Could you check a few things on this model? Use its own coordinates, in mm. Face numbers are marked on the shaded views. A direction names the side the tool comes from. Give positions to 0.01 mm unless a question says otherwise; leave off trailing zeros. Loops run counter-clockwise (first coordinate to the right, second up) from the corner with the lowest first, then second, coordinate; pieces in that order, holes last. Notation, with made-up numbers: (-13.75, 70.25) - (1.25, 70.25) arc R17 cw to (1.25, 84.25) - close; hole circle Ø7 at (62, 53). An arc over 180 degrees is marked (long way). Use CSV: the item, a comma, the result in double quotes.
from build123d import *

# Parameters (mm, degrees)
F_3_8_0_375_DIAMETER_HOLE1_D = 9.525
F_3_8_CLEARANCE_HOLE1_D      = 10.0838
CIRPATTERN1_COUNT            = 6


with BuildPart() as part:
    # Sketch1 → Revolve1 (revolve)
    with BuildSketch(Plane.XY):
        Polygon((-12.827, 0), (-50.8, 0), (-50.8, 12.7), (-19.05, 12.7), (-19.05, 38.1), (0, 38.1), (0, 0), (-9.525, 0), (-9.525, 2.54), (-12.827, 2.54), align=None)
    revolve(axis=Axis((0, 38.1, 0), (0, -1, 0)))

    # 3/8 (0.375) Diameter Hole1 (through all)
    with Locations(Plane(origin=(0, 38.1, 0), x_dir=(1, 0, 0), z_dir=(0, 1, 0))):
        with Locations((0, 0)):
            Hole(F_3_8_0_375_DIAMETER_HOLE1_D / 2)

    # Sketch3 → 1/2 NPT Tapped Hole1 (revolve, cut)
    with BuildSketch(Plane(origin=(0, 38.1, 0), x_dir=(0, 0, 1), z_dir=(1, 0, 0))):
        Polygon((0, 0), (0, 27.970543693), (8.9281, 22.606), (8.9281, 13.462), (9.479726792, 13.462), (9.8827971, 0), align=None)
    revolve(axis=Axis((0, 44.45, 0), (0, -1, 0)), mode=Mode.SUBTRACT)

    # 3/8 Clearance Hole1 (through all)
    with Locations(Plane(origin=(0, 12.7, 0), x_dir=(1, 0, 0), z_dir=(0, 1, 0))):
        with Locations((38.1, 0)):
            f_3_8_clearance_hole1 = Hole(F_3_8_CLEARANCE_HOLE1_D / 2)

    # CirPattern1: 3/8 Clearance Hole1 ×6 about axis
    cirpattern1_axis = Axis((0, 0, 0), (0, 1, 0))
    for i in range(1, CIRPATTERN1_COUNT):
        add(f_3_8_clearance_hole1.rotate(cirpattern1_axis, i * 360 / CIRPATTERN1_COUNT), mode=Mode.SUBTRACT)


solid = part.part
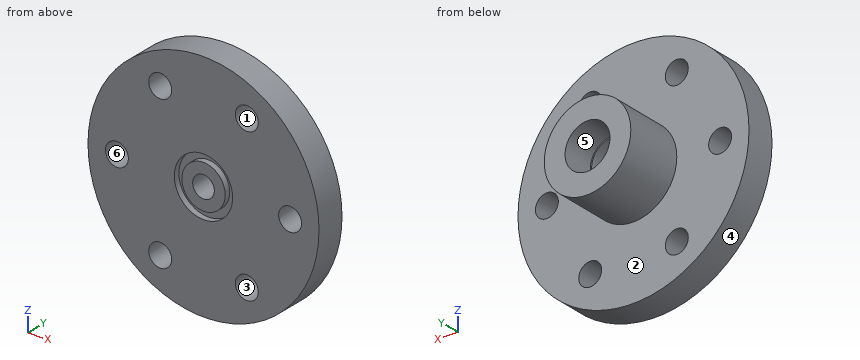
1) Which directions (+Z, -Z, +X, -X, +Y, -Y) give clear straight access to the entire face, cutting with the end or side of a thin tool? Please do the marked faces 5 and 6.
Answer below:
face 5,"+Y"
face 6,"+Y, -Y"
2) Suppose I cut it at B-B (x = 38.1). Please give me the cut outline in (y, z).
Answer below:
outline,"(0, -33.6) - (12.7, -33.6) - (12.7, -5.04) - (0, -5.04) - close; (0, 5.04) - (12.7, 5.04) - (12.7, 33.6) - (0, 33.6) - close"
3) We'd pull the mould along X, two halves only. Please class the marked faces 1, 2, 3 and 4: +X half, -X half, draft (parallel to the pull), parting line (faces both ways), or undercut.
Answer below:
face 1,"undercut"
face 2,"draft"
face 3,"undercut"
face 4,"parting line"
4) Suppose I cut it at D-D (z = -2). State how many separate pieces and enclosed holes the cut face has, plus the area to 3 significant figures.
Answer below:
separate pieces,"4"
enclosed holes,"0"
area,"1,440 mm2"
5) I'm going to push flat-ended pins straight in: P1, Ø9, axis at x = -38.1, z = 0, coming from the +Y side; P2, Ø11.5, axis at x = -19.05, z = 33, coming from the +Y side; P3, Ø1, axis at x = -9, y = 24, coming from the +Z side; P4, Ø1, axis at x = -2.5, y = 25, coming from the +Z side. Where does each tip first touch, or does it pass through?
Answer below:
P1,"passes through"
P2,"stops at y = 12.7"
P3,"stops at z = 17.05"
P4,"stops at z = 18.94"
6) I need wall thicknesses on line 1 along Z through (x, y) = (0, 17); line 2 along Z through (x, y) = (-19.05, 4); line 3 along Z through (x, y) = (0, 6). Which ranges of each line are inside material? Lowest first, please.
Answer below:
line 1,"z = -19.05 to -8.93, 8.93 to 19.05"
line 2,"z = -47.09 to -38.04, -27.95 to 27.95, 38.04 to 47.09"
line 3,"z = -50.8 to -4.76, 4.76 to 50.8"
7) Suppose I cut it at C-C (y = 27). Please give me the cut outline in (x, z), plus the area to 3 significant figures.
Answer below:
outline,"circle Ø38.1 at (0, 0); hole circle Ø19.1 at (0, 0)"
area,"854 mm2"
8) Suppose I cut it at A-A (z = 35). Please give me the cut outline in (x, y), plus the area to 3 significant figures.
Answer below:
outline,"(-36.82, 0) - (-23.68, 0) - (-23.68, 12.7) - (-36.82, 12.7) - close; (-14.42, 0) - (14.42, 0) - (14.42, 12.7) - (-14.42, 12.7) - close; (23.68, 0) - (36.82, 0) - (36.82, 12.7) - (23.68, 12.7) - close"
area,"700 mm2"
